from build123d import *

# Parameters (mm, degrees)
F0_W      = 57
F0_H      = 72
F0_R      = 2.25
F0_R_2    = 11.35
F1_DEPTH  = 6
F2_W      = 50
F2_H      = 3
F3_DEPTH  = 3
F4_W      = 50
F4_H      = 6
F5_DEPTH  = 1.5
F6_W      = 50
F6_H      = 6
F7_DEPTH  = 1.5
F8_W      = 12.50048
F8_H      = 66.124424
F9_DEPTH  = 3
F10_W     = 1.240771
F10_H     = 33.613906
F11_DEPTH = 3
F13_DEPTH = 54.5


with BuildPart() as f1:
    # F0 (on Top) → F1 (new body)
    with BuildSketch(Plane.XY):
        Rectangle(F0_W, F0_H)
        with Locations((-23.5, -32)):
            Circle(F0_R, mode=Mode.SUBTRACT)
        with BuildLine():
            Line((-25, -2.5), (-15.803481, -2.5))
            ThreePointArc((-15.803481, -2.5), (-11.313708, -11.313708), (-2.5, -15.803481))
            Line((-2.5, -15.803481), (-2.5, -25))
            Line((-2.5, -25), (-25, -25))
            Line((-25, -25), (-25, -2.5))
        make_face(mode=Mode.SUBTRACT)
        with Locations((23.5, -32)):
            Circle(F0_R, mode=Mode.SUBTRACT)
        with BuildLine():
            Line((15.803481, -2.5), (25, -2.5))
            Line((25, -2.5), (25, -25))
            Line((25, -25), (2.5, -25))
            Line((2.5, -25), (2.5, -15.803481))
            ThreePointArc((2.5, -15.803481), (11.313708, -11.313708), (15.803481, -2.5))
        make_face(mode=Mode.SUBTRACT)
        with BuildLine():
            Line((-2.5, 25), (-2.5, 15.803481))
            ThreePointArc((-2.5, 15.803481), (-11.313708, 11.313708), (-15.803481, 2.5))
            Line((-15.803481, 2.5), (-25, 2.5))
            Line((-25, 2.5), (-25, 25))
            Line((-25, 25), (-2.5, 25))
        make_face(mode=Mode.SUBTRACT)
        with Locations((-23.5, 32)):
            Circle(F0_R, mode=Mode.SUBTRACT)
        Circle(F0_R_2, mode=Mode.SUBTRACT)
        with BuildLine():
            Line((2.5, 25), (25, 25))
            Line((25, 25), (25, 2.5))
            Line((25, 2.5), (15.803481, 2.5))
            ThreePointArc((15.803481, 2.5), (11.313708, 11.313708), (2.5, 15.803481))
            Line((2.5, 15.803481), (2.5, 25))
        make_face(mode=Mode.SUBTRACT)
        with Locations((23.5, 32)):
            Circle(F0_R, mode=Mode.SUBTRACT)
    extrude(amount=F1_DEPTH)

    # F2 (on face) → F3 (join)
    with BuildSketch(Plane.XY.offset(6)):
        with Locations((0, -27.5)):
            Rectangle(F2_W, F2_H)
        with Locations((0, 27.5)):
            Rectangle(F2_W, F2_H)
    extrude(amount=F3_DEPTH)

    # F4 (on face) → F5 (join)
    with BuildSketch(Plane.XY.offset(9)):
        with Locations((0, -26)):
            Rectangle(F4_W, F4_H)
    extrude(amount=F5_DEPTH)

    # F6 (on face) → F7 (join)
    with BuildSketch(Plane.XY.offset(9)):
        with Locations((0, 26)):
            Rectangle(F6_W, F6_H)
    extrude(amount=F7_DEPTH)

    # F8 (on face) → F9 (cut)
    with BuildSketch(Plane.XY.offset(10.5)):
        Rectangle(F8_W, F8_H)
    extrude(amount=-F9_DEPTH, mode=Mode.SUBTRACT)

    # F10 (on face) → F11 (join)
    with BuildSketch(Plane.XY.offset(6)):
        with Locations((26.810841, 0)):
            Rectangle(F10_W, F10_H)
    extrude(amount=F11_DEPTH)

    # F12 (on face) → F13 (cut)
    with BuildSketch(Plane(origin=(-28.5, 0, 0), x_dir=(0, -1, 0), z_dir=(-1, 0, 0))):
        with BuildLine():
            Line((0, 6), (-26.086396, 6))
            ThreePointArc((-26.086396, 6), (-13.043198, 3.813688), (0, 6))
        make_face()
        with BuildLine():
            Line((25.915496, 6), (0, 6))
            ThreePointArc((0, 6), (12.957748, 3.843054), (25.915496, 6))
        make_face()
    extrude(amount=-F13_DEPTH, mode=Mode.SUBTRACT)


solid = f1.part
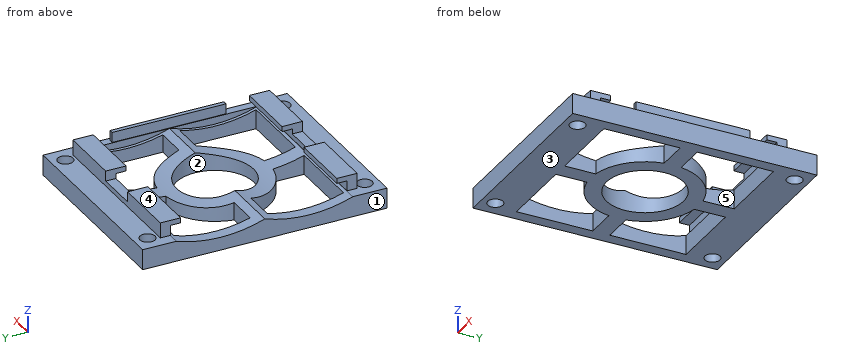
The model under review builds one solid part; all positions refer to its coordinate system, in mm. Face numbers are marked on the shaded views. A direction names the side the tool comes from. Round coordinates to 2 decimals unless told otherwise and drop trailing zeros. Order: outer loops, then holes, each group sorted by start corner. A loop starts at its lowest first (then second) coordinate and runs counter-clockwise, first axis right, second up. Notation, with made-up numbers: (11.5, 37) -> (40.5, 37) arc R22 ccw to (40.5, 73) -> close; hole circle Ø9 at (85, 72.5). An arc over 180 degrees is marked (long way). Return JSON: item names as keys, results as strings.
1. Take a section at A-A (z = 1.75). State how many separate pieces and enclosed holes the cut face has, then the cut area to 3 significant figures.
Answer block:
{"separate pieces": "1", "enclosed holes": "9", "area": "2,120 mm²"}
2. Take a section at B-B (y = 32). Write out the cut boundary in (x, z).
Answer block:
{"outline": "(-28.5, 0) -> (-25.75, 0) -> (-25.75, 6) -> (-28.5, 6) -> close; (-21.25, 0) -> (21.25, 0) -> (21.25, 6) -> (-21.25, 6) -> close; (25.75, 0) -> (28.5, 0) -> (28.5, 6) -> (25.75, 6) -> close"}
3. For L1, parallel to Y at x = -23.5, z = 2.7; L2, parallel to X at y = -24.5, z = 5.25; L3, parallel to Y at x = 17, z = 7.5, list the stretches that pass through material, from the lowest coordinate up. Write a range as [from, to].
Answer block:
{"L1": "y = [-36, -34.25], [-29.75, -25], [-2.5, 2.5], [25, 29.75], [34.25, 36]", "L2": "x = [-28.5, -25], [-2.5, 2.5], [25, 28.5]", "L3": "y = [-29, -26], [26, 29]"}
4. Insertion check: P1, Ø0.6, axis at x = 26.5, y = -1.5, coming from the +Z side; P2, Ø3.5, axis at y = -27, z = 9, coming from the -X side; P3, Ø10, axis at x = 8, y = 2.5, coming from the +Z side. Each pin has a flat end and moves straight along its axis. Give the tip position at first contact, or say it passes through.
Answer block:
{"P1": "stops at z = 9", "P2": "stops at x = -25", "P3": "stops at z = 6"}
5. For the marked faces 4 and 5, list the 3-axis set-ups (+Z, -Z, +X, -X, +Y, -Y) from which the entire face can be reached by the end or side of a thin tool; tool diameter is ignored.
Answer block:
{"face 4": "+Z, +X, -X, +Y, -Y", "face 5": "+Z, -Z"}
6. Take a section at C-C (x = 20). Write out the cut boundary in (y, z), then the cut area to 3 significant figures.
Answer block:
{"outline": "(-36, 0) -> (-25, 0) -> (-25, 5.7) arc R40 cw to (-25.92, 6) -> (-26, 6) -> (-26, 9) -> (-23, 9) -> (-23, 10.5) -> (-29, 10.5) -> (-29, 6) -> (-36, 6) -> close; (-2.5, 0) -> (2.5, 0) -> (2.5, 5.23) arc R40 cw to (0, 6) arc R40 cw to (-2.5, 5.23) -> close; (23, 9) -> (26, 9) -> (26, 6) -> (26.09, 6) arc R40 cw to (25, 5.64) -> (25, 0) -> (36, 0) -> (36, 6) -> (29, 6) -> (29, 10.5) -> (23, 10.5) -> close", "area": "196 mm²"}
7. Take a section at D-D (y = 6). Write out the cut boundary in (x, z).
Answer block:
{"outline": "(-28.5, 0) -> (-25, 0) -> (-25, 4.44) -> (-28.5, 4.44) -> close; (-14.83, 0) -> (-9.63, 0) -> (-9.63, 4.44) -> (-14.83, 4.44) -> close; (9.63, 0) -> (14.83, 0) -> (14.83, 4.44) -> (9.63, 4.44) -> close; (25, 0) -> (28.5, 0) -> (28.5, 6) -> (27.43, 6) -> (27.43, 9) -> (26.19, 9) -> (26.19, 6) -> (26, 6) -> (26, 4.44) -> (25, 4.44) -> close"}
8. The part is to be moulded in two halves that separate along X. For the marked faces 1, 2 and 3, say which applies: +X half, -X half, draft (parallel to the pull), parting line (faces both ways), or undercut.
Answer block:
{"face 1": "-X half", "face 2": "undercut", "face 3": "draft"}
